Job drawing, mm, ordinate dimensions from the low corner. One solid piece. Coordinates: 2 decimals unless noted, no trailing zeros. Write each loop counter-clockwise with the first axis right and the second up, starting at its lowest first coordinate (ties: lowest second). Pieces come first, ordered by that corner, then holes. Notation, with made-up numbers: (1.25, 20) - (7.25, 20) arc R28 ccw to (7.25, 40) - close; hole circle Ø1 at (10, 67). An arc over 180 degrees is marked (long way). Put each result on its own line as item: value. Start each with the question number.
1. Saw through at B-B, the plane y = 2.4. Write the cut outline in (x, z).
2. Saw through at A-A, the plane x = 86. Write the cut outline in (y, z).
3. Drop flat-ended pins along their axis: P1, Ø1.5, axis at y = 2, z = 3.5, coming from the -X side; P2, Ø2.5, axis at x = 53.85, z = 6, coming from the +Y side. Give the stop position or say it passes through.
4. Saw through at C-C, the plane z = 6. Write the cut outline in (x, y), plus the area to 3 significant figures.
5. Drill centre lines: L1, parallel to X at y = 0.8, z = 6; L2, parallel to X at y = 0.3, z = 6.75; L3, parallel to Z at x = 6.4, y = 1.8. Where is each one in solid material? Low to high. Write a range as from..to.
6. Saw through at D-D, the plane x = 73.5. Write the cut outline in (y, z), plus the area to 3 significant figures.
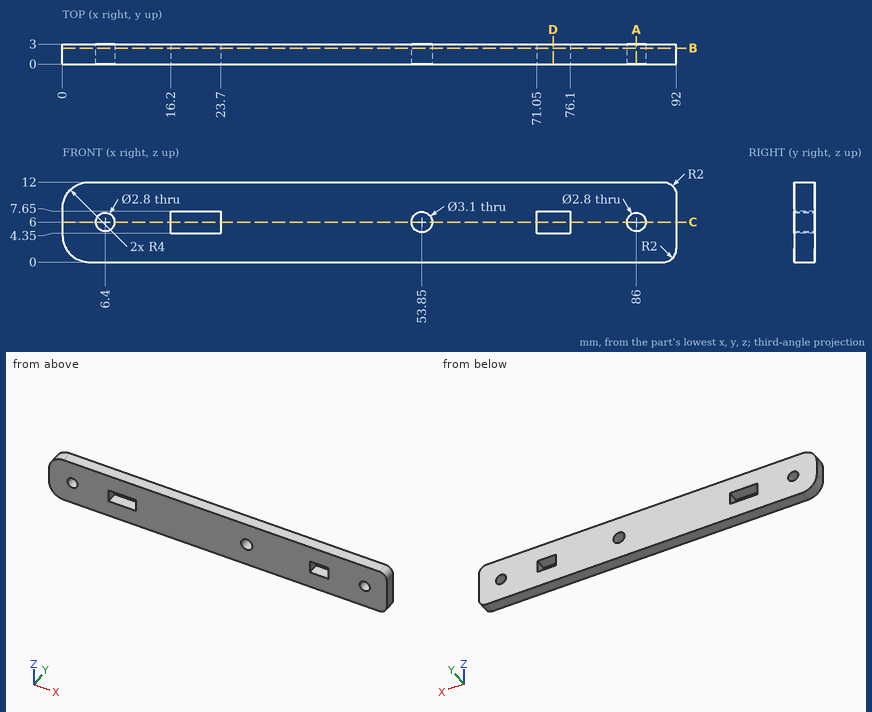
Final values:
1. outline: (0, 4) arc R4 ccw to (4, 0) - (90, 0) arc R2 ccw to (92, 2) - (92, 10) arc R2 ccw to (90, 12) - (4, 12) arc R4 ccw to (0, 8) - close; hole circle Ø2.8 at (6.4, 6); hole (16.2, 4.35) - (23.7, 4.35) - (23.7, 7.65) - (16.2, 7.65) - close; hole circle Ø3.1 at (53.85, 6); hole (71.05, 4.35) - (76.1, 4.35) - (76.1, 7.65) - (71.05, 7.65) - close; hole circle Ø2.8 at (86, 6)
2. outline: (0, 0) - (3, 0) - (3, 4.6) - (0, 4.6) - close; (0, 7.4) - (3, 7.4) - (3, 12) - (0, 12) - close
3. P1: stops at x = 0
3. P2: passes through
4. outline: (0, 0) - (5, 0) - (5, 3) - (0, 3) - close; (7.8, 0) - (16.2, 0) - (16.2, 3) - (7.8, 3) - close; (23.7, 0) - (52.3, 0) - (52.3, 3) - (23.7, 3) - close; (55.4, 0) - (71.05, 0) - (71.05, 3) - (55.4, 3) - close; (76.1, 0) - (84.6, 0) - (84.6, 3) - (76.1, 3) - close; (87.4, 0) - (92, 0) - (92, 3) - (87.4, 3) - close
4. area: 212 mm²
5. L1: x = 0..5, 7.8..16.2, 23.7..52.3, 55.4..71.05, 76.1..84.6, 87.4..92
5. L2: x = 0..5.22, 7.58..16.2, 23.7..52.49, 55.21..71.05, 76.1..84.82, 87.18..92
5. L3: z = 0..4.6, 7.4..12
6. outline: (0, 0) - (3, 0) - (3, 4.35) - (0, 4.35) - close; (0, 7.65) - (3, 7.65) - (3, 12) - (0, 12) - close
6. area: 26.1 mm²
